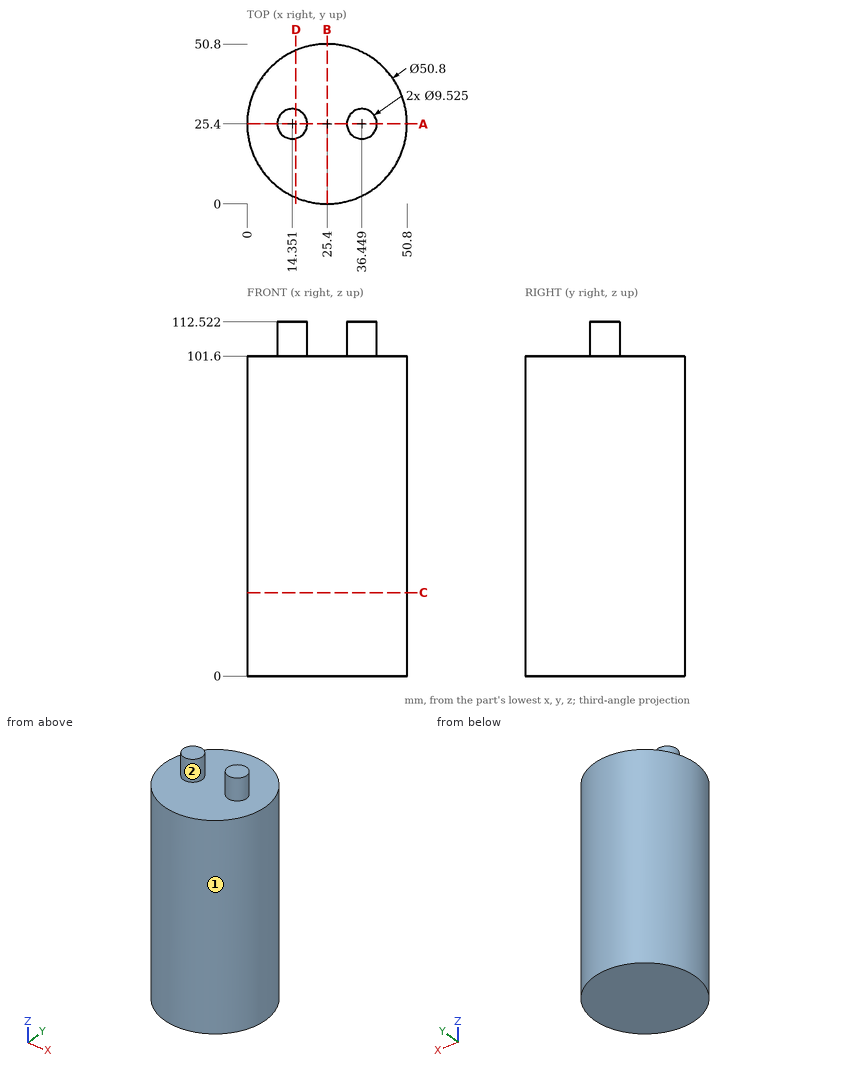
Answer from the drawing. Dimensions are ordinates in mm from the lowest x, y and z of the part. A direction names the side the tool comes from. Coordinates: 2 decimals unless noted, no trailing zeros. Loops run counter-clockwise (first coordinate to the right, second up) from the corner with the lowest first, then second, coordinate; pieces in that order, holes last.
Q1. Each of these flat-tipped pins is pushed along its axis until it touches: pin 1 Ø3 at (x, y) = (17.5, 18) entering from +Z; pin 2 Ø4 at (y, z) = (39.5, 50.5) entering from -X; pin 3 Ø1 at (y, z) = (15, 99) entering from -X. Where does it stop, or does it pass through?
Q2. The part is cut by section C-C on z = 26.5. Write down the section's boundary in (x, y).
Q3. The part is cut by section A-A on y = 25.4. Write down the section's boundary in (x, z).
Q4. The part is cut by section B-B on x = 25.4. Write down the section's boundary in (y, z), and give its area (3 significant figures).
Q5. The part is cut by section D-D on x = 15.5. Write down the section's boundary in (y, z).
Q6. Which of the six approach directions +Z, -Z, +X, -X, +Y, -Y give full straight-line access (tool end or side, diameter ignored) to the marked faces 1 and 2?
Q7. Consider probe 1 along Z at (x, y) = (19, 12); probe 2 along Y at (x, z) = (25, 100.5); probe 3 along X at (y, z) = (3.5, 13.5). Determine where each line is inside the solid, lowest interval first.
Results below:
1. pin 1: stops at z = 101.6
1. pin 2: stops at x = 3.07
1. pin 3: stops at x = 2.01
2. outline: circle Ø50.8 at (25.4, 25.4)
3. outline: (0, 0) - (50.8, 0) - (50.8, 101.6) - (41.21, 101.6) - (41.21, 112.52) - (31.69, 112.52) - (31.69, 101.6) - (19.11, 101.6) - (19.11, 112.52) - (9.59, 112.52) - (9.59, 101.6) - (0, 101.6) - close
4. outline: (0, 0) - (50.8, 0) - (50.8, 101.6) - (0, 101.6) - close
4. area: 5,160 mm2
5. outline: (2.01, 0) - (48.79, 0) - (48.79, 101.6) - (30.02, 101.6) - (30.02, 112.52) - (20.78, 112.52) - (20.78, 101.6) - (2.01, 101.6) - close
6. face 1: +Z, -Z
6. face 2: +Z
7. probe 1: z = 0 to 101.6
7. probe 2: y = 0 to 50.8
7. probe 3: x = 12.53 to 38.27
